```python
from build123d import *

# Parameters (mm, degrees)
SKETCH1_R           = 7.9375
BASE_EXTRUDE_DEPTH  = 101.6
BOSS_EXTRUDE1_DEPTH = 9.525
SKETCH3_R           = 7.9375
BOSS_EXTRUDE2_DEPTH = 9.525


with BuildPart() as part:
    # Sketch1 → Base-Extrude (new body)
    with BuildSketch(Plane.XY):
        Circle(SKETCH1_R)
    extrude(amount=BASE_EXTRUDE_DEPTH)

    # Sketch2 → Boss-Extrude1 (add)
    with BuildSketch(Plane.XY.offset(101.6)):
        Polygon((12.7, -7.332348419), (12.7, 7.332348419), (0, 14.664696837), (-12.7, 7.332348419), (-12.7, -7.332348419), (0, -14.664696837), align=None)
    extrude(amount=BOSS_EXTRUDE1_DEPTH)

    # Sketch3 → Boss-Extrude2 (add)
    with BuildSketch(Plane.XY.offset(111.125)):
        Circle(SKETCH3_R)
    extrude(amount=BOSS_EXTRUDE2_DEPTH)


solid = part.part
```
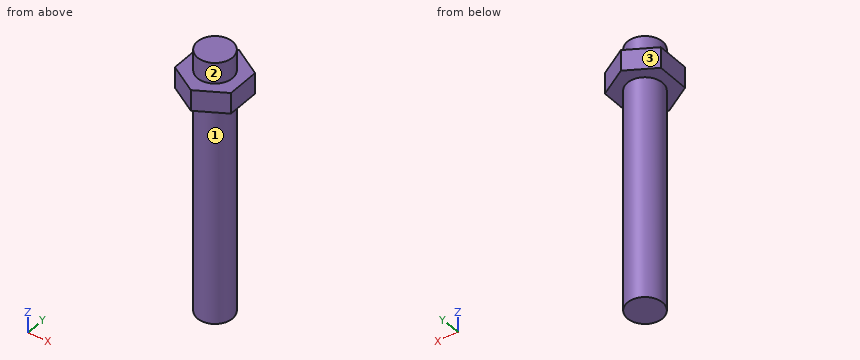
Model file for the job. Use its own axes, mm. Face numbers are marked on the shaded views. A direction names the side the tool comes from. Give positions to 0.01 mm unless a question says otherwise; leave off trailing zeros. Loops run counter-clockwise (first coordinate to the right, second up) from the corner with the lowest first, then second, coordinate; pieces in that order, holes last. Notation, with made-up numbers: (-24, 21.5) -> (-1, 21.5) arc R27 cw to (-1, 42.5) -> close; hole circle Ø3 at (-5.5, -36.5). An arc over 180 degrees is marked (long way). Write each question's results on one line, items separated by ' | '.
(1) Cut at B-B on x = -2.75. List the corners of the cut face in (y, z) (3 decimals).
Geometry results:
outline: (-13.077, 101.6) -> (-7.446, 101.6) -> (-7.446, 0) -> (7.446, 0) -> (7.446, 101.6) -> (13.077, 101.6) -> (13.077, 111.125) -> (7.446, 111.125) -> (7.446, 120.65) -> (-7.446, 120.65) -> (-7.446, 111.125) -> (-13.077, 111.125) -> close
(2) Probe line 1 along Z through (x, y) = (11, 7) (3 decimals); line 2 along Y through (x, z) = (-3, 101.5); line 3 along Y through (x, z) = (-0.25, 51). List the from-to ranges inside material, lowest first.
Geometry results:
line 1: z = 101.6 to 111.125 | line 2: y = -7.35 to 7.35 | line 3: y = -7.93 to 7.93
(3) Cut at C-C on z = 33.5. List the corners of the cut face in (x, y) (1 decimal), and give its area (3 significant figures).
Geometry results:
outline: circle Ø15.9 at (0, 0) | area: 198 mm²
(4) Tool access for the marked faces 1, 2 and 3: list every direction of +Z, -Z, +X, -X, +Y, -Y with a clear straight run to the whole face (end or side of a thin tool).
Geometry results:
face 1: -Z | face 2: +Z | face 3: +Z, -Z, -X, +Y
(5) Flat gauge pins, fed straight in: pin 1 Ø2 at (x, z) = (7, 55) entering from +Y; pin 2 Ø3 at (y, z) = (-0.5, 34) entering from +X; pin 3 Ø1.5 at (y, z) = (-10.5, 90.5) entering from +X; pin 4 Ø4 at (x, y) = (8.5, 7.5) entering from +Z (3 decimals). Where does each tip first touch, or does it go through?
Geometry results:
pin 1: stops at y = 5.2 | pin 2: stops at x = 7.94 | pin 3: passes through | pin 4: stops at z = 111.125
(6) Cut at D-D on y = 9.5. List the corners of the cut face in (x, z) (3 decimals).
Geometry results:
outline: (-8.946, 101.6) -> (8.946, 101.6) -> (8.946, 111.125) -> (-8.946, 111.125) -> close
